from build123d import *

# Parameters (mm, degrees)
BOSS_EXTRUDE1_DEPTH = 18.288
FILLET1_R           = 6.35


with BuildPart() as part:
    # Sketch1 → Boss-Extrude1 (new body)
    with BuildSketch(Plane(origin=(0, 0, 0), x_dir=(0, 0, -1), z_dir=(1, 0, 0))):
        with BuildLine():
            Line((-166.973473818, -57.646230654), (123.785960254, -57.646230654))
            ThreePointArc((123.785960254, -57.646230654), (128.276088314, -55.786358715), (130.135960254, -51.296230654))
            Line((130.135960254, -51.296230654), (130.135960254, 12.203769346))
            ThreePointArc((130.135960254, 12.203769346), (128.276088314, 16.693897406), (123.785960254, 18.553769346))
            Line((123.785960254, 18.553769346), (66.971101736, 18.553769346))
            ThreePointArc((66.971101736, 18.553769346), (66.636426055, 18.5449437), (66.302680683, 18.518491295))
            Line((66.302680683, 18.518491295), (-167.641894871, -6.244828564))
            ThreePointArc((-167.641894871, -6.244828564), (-171.694012648, -8.31231457), (-173.323473818, -12.559550513))
            Line((-173.323473818, -12.559550513), (-173.323473818, -51.296230654))
            ThreePointArc((-173.323473818, -51.296230654), (-171.463601879, -55.786358715), (-166.973473818, -57.646230654))
        make_face()
    extrude(amount=BOSS_EXTRUDE1_DEPTH)

    # Fillet1
    fillet1_edges = [part.edges().sort_by_distance(p)[0] for p in [
        (18.288, -8.31231457, 171.694012648),
        (0, -19.546230654, -130.135960254),
        (0, -55.786358715, -128.276088314),
        (0, -57.646230654, 21.593756782),
        (0, -55.786358715, 171.463601879),
        (0, -31.927890584, 173.323473818),
        (0, -8.31231457, 171.694012648),
        (0, 6.136831366, 50.669607094),
        (0, 18.5449437, -66.636426055),
        (18.288, -31.927890584, 173.323473818),
        (18.288, -55.786358715, 171.463601879),
        (18.288, -57.646230654, 21.593756782),
        (18.288, -55.786358715, -128.276088314),
        (18.288, -19.546230654, -130.135960254),
        (18.288, 16.693897406, -128.276088314),
        (18.288, 18.553769346, -95.378530995),
        (18.288, 18.5449437, -66.636426055),
        (18.288, 6.136831366, 50.669607094),
        (0, 18.553769346, -95.378530995),
        (0, 16.693897406, -128.276088314),
    ]]
    fillet(fillet1_edges, radius=FILLET1_R)


solid = part.part
The model under review builds one solid part; all positions refer to its coordinate system, in mm. Round coordinates to 2 decimals unless told otherwise and drop trailing zeros. Write each loop counter-clockwise with the first axis right and the second up, starting at its lowest first coordinate (ties: lowest second). Pieces come first, ordered by that corner, then holes. Notation, with made-up numbers: M 87,49 L 117,49 A32 ccw 117,76 Z; hole C 48,-34 d11. An arc over 180 degrees is marked long. Use a Markdown table: item, result. Add a question column.
Q1. Insertion check: pin 1 (3 mm diameter, centred on x = 14, z = 23, fed in from -Y); pin 2 (8 mm diameter, centred on x = 12.5, y = -33.5, fed in from +Z); pin 3 (1.5 mm diameter, centred on x = 3.5, z = -99, fed in from +Y). Each pin has a flat end and moves straight along its axis. Give the tip position at first contact, or say it passes through.
Q2. To check wall thickness, follow line 1 (Y direction, x = 7.5, z = 37.5); line 2 (Y direction, x = 5.5, z = 29.5); line 3 (Z direction, x = 3.25, y = -29). State the ranges of each line that lie inside material, in increasing order.
Q3. We need section A-A, the plane z = -74.5. State the section outline as (x, y) points, plus the area to 3 significant figures.
Q4. We need section B-B, the plane x = 9. State the section outline as (y, z) points.
Findings below:
| question | item | result |
|---|---|---|
| 1 | pin 1 | stops at y = -57.62 |
| 1 | pin 2 | stops at z = 173.32 |
| 1 | pin 3 | stops at y = 18.2 |
| 2 | line 1 | y = -57.65 to 7.53 |
| 2 | line 2 | y = -57.59 to 8.32 |
| 2 | line 3 | z = -129.33 to 172.52 |
| 3 | outline | M 0,-51.3 A6.35 ccw 6.35,-57.65 L 11.94,-57.65 A6.35 ccw 18.29,-51.3 L 18.29,12.2 A6.35 ccw 11.94,18.55 L 6.35,18.55 A6.35 ccw 0,12.2 Z |
| 3 | area | 1,360 mm² |
| 4 | outline | M -57.65,-123.79 A6.35 ccw -51.3,-130.14 L 12.2,-130.14 A6.35 ccw 18.55,-123.79 L 18.55,-66.97 A6.35 ccw 18.52,-66.3 L -6.24,167.64 A6.35 ccw -12.56,173.32 L -51.3,173.32 A6.35 ccw -57.65,166.97 Z |
